Autodesk Inventor part; units mm, degrees
ref_plane "YZ Plane" through (0, 0, 0) normal (1, 0, 0) x (0, 1, 0)
ref_plane "XZ Plane" through (0, 0, 0) normal (0, 1, 0) x (-1, 0, 0)
ref_plane "XY Plane" through (0, 0, 0) normal (0, 0, 1) x (1, 0, 0)
sketch "Sketch1" plane through (0, 0, 0) normal (0, 0, 1) x (1, 0, 0)
  circle A0 centre (0, 0) radius 3.175
  dimension "d0" = 6.35
extrude "Extrusion1" add sketch "Sketch1" along normal blind 63.5
sketch "Sketch2" plane through (0, 0, 63.5) normal (0, 0, 1) x (1, 0, 0)
  circle A0 centre (0, 0) radius 3.175
  line L0 (3.2079, 5.5562) -> (6.4158, 0)
  line L1 (6.4158, 0) -> (3.2079, -5.5562)
  line L2 (3.2079, -5.5562) -> (-3.2079, -5.5562)
  line L3 (-3.2079, -5.5562) -> (-6.4158, 0)
  line L4 (-6.4158, 0) -> (-3.2079, 5.5562)
  line L5 (-3.2079, 5.5562) -> (3.2079, 5.5562)
  dimension "d4" = 11.1125
extrude "Extrusion2" add sketch "Sketch2" along normal blind 4.7625 contours A0 | L0 L1 L2 L3 L4 L5
fillet "Fillet1" radius 0.254 12 edges at (4.8119, 2.7781, 68.2625) (0, 5.5562, 68.2625) (-4.8119, 2.7781, 68.2625) (-4.8119, -2.7781, 68.2625) (0, -5.5562, 68.2625) (4.8119, -2.7781, 68.2625) (4.8119, -2.7781, 63.5) (4.8119, 2.7781, 63.5) (0, 5.5562, 63.5) (-4.8119, 2.7781, 63.5) (-4.8119, -2.7781, 63.5) (0, -5.5562, 63.5)
thread "Thread1"
properties part number "Deck_Bolt"
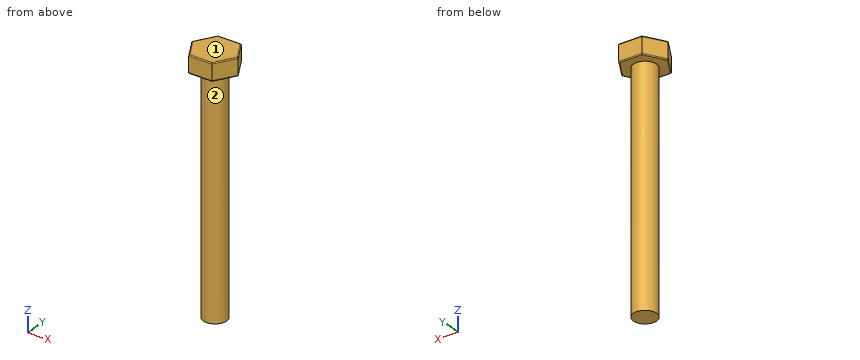
Design review of the part built by this model. Coordinates are the model's own, in mm. Face numbers are marked on the shaded views. A direction names the side the tool comes from. Coordinates: 2 decimals unless noted, no trailing zeros. Order: outer loops, then holes, each group sorted by start corner. A loop starts at its lowest first (then second) coordinate and runs counter-clockwise, first axis right, second up. Notation, with made-up numbers: (64.25, 57.25) -> (72.25, 57.25) arc R23 ccw to (72.25, 95.25) -> close; hole circle Ø7 at (-19.5, 80). An arc over 180 degrees is marked (long way). One line per item, written item: value. Start each with the question number.
Q1. Insertion check: pin 1 Ø2 at (y, z) = (2, 54.5) entering from -X; pin 2 Ø3 at (y, z) = (1, 9.5) entering from -X (3 decimals); pin 3 Ø2 at (y, z) = (3, 42.5) entering from +X. Each pin has a flat end and moves straight along its axis. Give the tip position at first contact, or say it passes through.
Q2. Take a section at B-B, the plane z = 14. State the section outline as (x, y) points (3 decimals), then the cut area to 3 significant figures.
Q3. For probe 1 along Z at (x, y) = (-2.5, -2.5); probe 2 along Y at (x, z) = (0, 6) (3 decimals); probe 3 along X at (y, z) = (-1.5, 48), list the stretches that pass through material, from the lowest coordinate up.
Q4. Tool access review of the marked faces 1 and 2: name each direction out of +Z, -Z, +X, -X, +Y, -Y from which nothing blocks a thin tool from reaching the whole face with its end or side.
Values follow:
1. pin 1: stops at x = -3.01
1. pin 2: stops at x = -3.175
1. pin 3: stops at x = 2.47
2. outline: circle Ø6.35 at (0, 0)
2. area: 31.7 mm2
3. probe 1: z = 63.5 to 68.26
3. probe 2: y = -3.175 to 3.175
3. probe 3: x = -2.8 to 2.8
4. face 1: +Z, +X, -X, +Y, -Y
4. face 2: -Z
